The listing builds one solid part. Answer for the finished solid, in the listing's coordinates (mm). Face numbers are marked on the shaded views. A direction names the side the tool comes from. Round coordinates to 2 decimals unless told otherwise and drop trailing zeros. Write each loop counter-clockwise with the first axis right and the second up, starting at its lowest first coordinate (ties: lowest second). Pieces come first, ordered by that corner, then holes. Notation, with made-up numbers: (21, 57) - (49, 57) arc R27 cw to (49, 75) - close; hole circle Ø11 at (37, 63). An arc over 180 degrees is marked (long way). Return JSON: item names as keys, results as strings. Group by question number.
(1) Section D-D, the plane z = 7.75 is taken. Write down the section's boundary in (x, y), then the cut area to 3 significant figures.
(2) Section B-B, the plane z = 3.5 is taken. Write down the section's boundary in (x, y), then the cut area to 3 significant figures.
(3) This flat-tipped pin is pushed along its axis until it touches: pin 1 (2.5 mm diameter, centred on x = -39, y = 3, fed in from -Z). Where does it stop, or does it pass through?
(4) Which of the six approach directions +Z, -Z, +X, -X, +Y, -Y give full straight-line access (tool end or side, diameter ignored) to the marked faces 4, 5, 6 and 7?
(5) Section C-C, the plane y = 13.5 is taken. Write down the section's boundary in (x, z) (3 decimals).
(6) Section A-A, the plane x = -46.5 is taken. Write down the section's boundary in (y, z), then the cut area to 3 significant figures.
(7) Find the intervals of material crossed by line 1 along X through (y, z) = (11.25, -8.5) (3 decimals); line 2 along X through (y, z) = (13, 2.5); line 3 along Y through (x, z) = (-40.75, 0), in increasing order. Write a range as [from, to].
(8) Determine the mould class of the marked faces 1, 2 and 3 for opening direction Z: +Z half, -Z half, draft (parallel to the pull), parting line (faces both ways), or undercut.
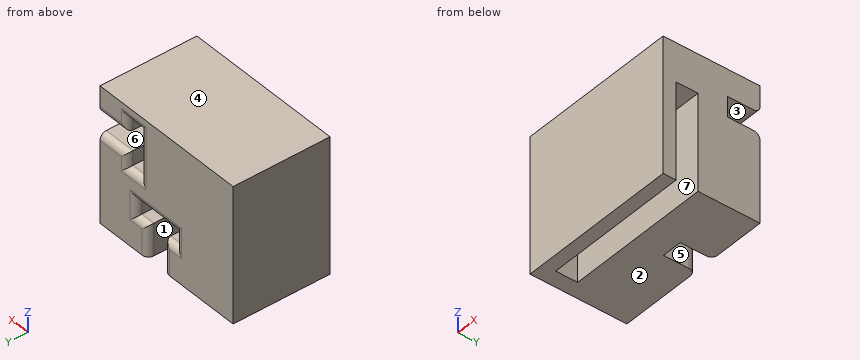
```python
from build123d import *

# Parameters (mm, degrees)
SKETCH1_W           = 25
SKETCH1_H           = 21
BOSS_EXTRUDE1_DEPTH = 15
SKETCH2_W           = 15
SKETCH2_H           = 3.4
CUT_EXTRUDE1_DEPTH  = 22.6
CUT_EXTRUDE2_DEPTH  = 5
FILLET1_R           = 1


with BuildPart() as part:
    # Sketch1 → Boss-Extrude1 (new body)
    with BuildSketch(Plane(origin=(0, 0, 0), x_dir=(1, 0, 0), z_dir=(0, 1, 0))):
        Rectangle(SKETCH1_W, SKETCH1_H)
    extrude(amount=BOSS_EXTRUDE1_DEPTH)

    # Sketch2 → Cut-Extrude1 (cut)
    with BuildSketch(Plane.ZY.offset(12.5)):
        with Locations((-3, 3.7)):
            Rectangle(SKETCH2_W, SKETCH2_H)
    extrude(amount=-CUT_EXTRUDE1_DEPTH, mode=Mode.SUBTRACT)

    # Sketch3 → Cut-Extrude2 (cut)
    with BuildSketch(Plane(origin=(0, 15, 0), x_dir=(1, 0, 0), z_dir=(0, 1, 0))):
        Polygon((-4.85, -0.925), (-4.85, -8.575), (-7.5, -8.575), (-7.5, -6.325), (-12.5, -6.325), (-12.5, -3.175), (-7.5, -3.175), (-7.5, -0.925), align=None)
        Polygon((-3.575, 10.5), (-3.575, 5.5), (-5.825, 5.5), (-5.825, 2.85), (1.825, 2.85), (1.825, 5.5), (-0.425, 5.5), (-0.425, 10.5), align=None)
    extrude(amount=-CUT_EXTRUDE2_DEPTH, mode=Mode.SUBTRACT)

    # Fillet1
    fillet1_edges = [part.edges().sort_by_distance(p)[0] for p in [
        (-6.175, 15, 0.925),
        (-7.5, 15, 2.05),
        (-10, 15, 3.175),
        (-10, 15, 6.325),
        (-7.5, 15, 7.45),
        (-6.175, 15, 8.575),
        (-4.85, 15, 4.75),
        (-3.575, 15, -8),
        (-4.7, 15, -5.5),
        (-5.825, 15, -4.175),
        (-2, 15, -2.85),
        (1.825, 15, -4.175),
        (0.7, 15, -5.5),
        (-0.425, 15, -8),
    ]]
    fillet(fillet1_edges, radius=FILLET1_R)


with BuildPart() as body_2:
    # Mirror2: mirrored copy
    add(part.part.mirror(Plane.ZY.offset(22.5)))


solid = body_2.part
```
Working result:
{
 "1": {"outline": "(-57.5, 0) - (-32.5, 0) - (-32.5, 15) - (-36.5, 15) arc R1 ccw to (-37.5, 14) - (-37.5, 10) - (-40.15, 10) - (-40.15, 14) arc R1 ccw to (-41.15, 15) - (-57.5, 15) - close", "area": "361 mm^2"},
 "2": {"outline": "(-57.5, 0) - (-32.5, 0) - (-32.5, 2) - (-55.1, 2) - (-55.1, 5.4) - (-32.5, 5.4) - (-32.5, 10) - (-40.15, 10) - (-40.15, 14) arc R1 ccw to (-41.15, 15) - (-57.5, 15) - close", "area": "260 mm^2"},
 "3": {"pin 1": "stops at z = -10.5"},
 "4": {"face 4": "+Z, +X, -X, +Y, -Y", "face 5": "-Z, +Y", "face 6": "+X, +Y", "face 7": "-Z, +X"},
 "5": {"outline": "(-57.5, -10.5) - (-44.575, -10.5) - (-44.575, -5.5) - (-46.825, -5.5) - (-46.825, -2.85) - (-39.175, -2.85) - (-39.175, -5.5) - (-41.425, -5.5) - (-41.425, -10.5) - (-32.5, -10.5) - (-32.5, 3.175) - (-37.5, 3.175) - (-37.5, 0.925) - (-40.15, 0.925) - (-40.15, 8.575) - (-37.5, 8.575) - (-37.5, 6.325) - (-32.5, 6.325) - (-32.5, 10.5) - (-57.5, 10.5) - close"},
 "6": {"outline": "(0, -10.5) - (2, -10.5) - (2, 4.5) - (5.4, 4.5) - (5.4, -10.5) - (15, -10.5) - (15, -6.5) arc R1 ccw to (14, -5.5) - (10, -5.5) - (10, -2.85) - (14, -2.85) arc R1 ccw to (15, -1.85) - (15, 10.5) - (0, 10.5) - close", "area": "250 mm^2"},
 "7": {"line 1": "x = [-57.5, -44.575], [-41.425, -32.5]", "line 2": "x = [-57.5, -40.15], [-37.5, -32.5]", "line 3": "y = [0, 2], [5.4, 15]"},
 "8": {"face 1": "draft", "face 2": "-Z half", "face 3": "undercut"}
}
